from build123d import *

# Parameters (mm, degrees)
DODANIE_WYCI_GNI_CIE1_DEPTH = 40
ZAOKR_GLENIE1_R             = 20
SZKIC2_R                    = 12
WYTNIJ_WYCI_GNI_CIE1_DEPTH  = 725.630250542
SZKIC3_R                    = 8.15
WYTNIJ_WYCI_GNI_CIE2_DEPTH  = 725.630250542
SZKIC5_R                    = 14
DODANIE_WYCI_GNI_CIE2_DEPTH = 40
SZKIC6_W                    = 20
SZKIC6_H                    = 55
WYTNIJ_WYCI_GNI_CIE4_DEPTH  = 778.890737829
SZKIC4_R                    = 1.65
WYTNIJ_WYCI_GNI_CIE5_DEPTH  = 10
SFAZOWANIE1_SIZE            = 0.5
SFAZOWANIE2_SIZE            = 1


with BuildPart() as part:
    # Szkic1 → Dodanie-wyciągnięcie1 (new body)
    with BuildSketch(Plane.XY):
        Polygon((0, 0), (30, 0), (30, 670), (153, 670), (153, 0), (183, 0), (183, 700), (110, 700), (30, 700), (0, 700), align=None)
    extrude(amount=DODANIE_WYCI_GNI_CIE1_DEPTH)

    # Zaokrąglenie1
    zaokr_glenie1_edges = [part.edges().sort_by_distance(p)[0] for p in [
        (168, 0, 0),
        (168, 0, 40),
        (15, 0, 0),
        (15, 0, 40),
    ]]
    fillet(zaokr_glenie1_edges, radius=ZAOKR_GLENIE1_R - 0.0001)  # a hair under: the kernel refuses the full size

    # Szkic2 → Wytnij-wyciągnięcie1 (cut, through all)
    with BuildSketch(Plane.ZY):
        with Locations((20, 20)):
            Circle(SZKIC2_R)
    extrude(amount=-WYTNIJ_WYCI_GNI_CIE1_DEPTH, mode=Mode.SUBTRACT)

    # Szkic3 → Wytnij-wyciągnięcie2 (cut, through all)
    with BuildSketch(Plane(origin=(183, 0, 0), x_dir=(0, 0, -1), z_dir=(1, 0, 0))):
        with Locations(Location((-20, 70, 0), (0, 0, 90))):
            Circle(SZKIC3_R)
    extrude(amount=-WYTNIJ_WYCI_GNI_CIE2_DEPTH, mode=Mode.SUBTRACT)

    # Szkic5 → Dodanie-wyciągnięcie2 (add)
    with BuildSketch(Plane(origin=(0, 0, 0), x_dir=(-1, 0, 0), z_dir=(0, 0, -1))):
        with BuildLine():
            Line((-183, 700), (0, 700))
            Line((0, 700), (-74.84618459, 749.952964399))
            ThreePointArc((-74.84618459, 749.952964399), (-91.5, 755), (-108.15381541, 749.952964399))
            Line((-108.15381541, 749.952964399), (-183, 700))
        make_face()
        with Locations((-91.5, 725)):
            Circle(SZKIC5_R, mode=Mode.SUBTRACT)
    extrude(amount=-DODANIE_WYCI_GNI_CIE2_DEPTH)

    # Szkic6 → Wytnij-wyciągnięcie4 (cut, through all)
    with BuildSketch(Plane(origin=(183, 0, 0), x_dir=(0, 0, -1), z_dir=(1, 0, 0))):
        with Locations((-20, 727.5)):
            Rectangle(SZKIC6_W, SZKIC6_H)
    extrude(amount=-WYTNIJ_WYCI_GNI_CIE4_DEPTH, mode=Mode.SUBTRACT)

    # Szkic4 → Wytnij-wyciągnięcie5 (cut)
    with BuildSketch(Plane.ZY.offset(-153)):
        with Locations(Location((20, 657.5, 0), (0, 0, 270))):
            Circle(SZKIC4_R)
        with Locations(Location((20, 597.5, 0), (0, 0, 270))):
            Circle(SZKIC4_R)
        with Locations(Location((20, 537.5, 0), (0, 0, 270))):
            Circle(SZKIC4_R)
        with Locations(Location((20, 477.5, 0), (0, 0, 270))):
            Circle(SZKIC4_R)
        with Locations(Location((20, 417.5, 0), (0, 0, 270))):
            Circle(SZKIC4_R)
    extrude(amount=-WYTNIJ_WYCI_GNI_CIE5_DEPTH, mode=Mode.SUBTRACT)

    # Sfazowanie1
    sfazowanie1_edges = [part.edges().sort_by_distance(p)[0] for p in [
        (153, 659.15, 20),
        (153, 599.15, 20),
        (153, 539.15, 20),
        (153, 479.15, 20),
        (153, 419.15, 20),
    ]]
    chamfer(sfazowanie1_edges, length=SFAZOWANIE1_SIZE)

    # Sfazowanie2
    sfazowanie2_edges = [part.edges().sort_by_distance(p)[0] for p in [
        (30, 20, 8),
        (183, 20, 8),
        (153, 20, 8),
        (0, 20, 8),
        (0, 61.85, 20),
        (30, 61.85, 20),
        (153, 61.85, 20),
        (183, 61.85, 20),
    ]]
    chamfer(sfazowanie2_edges, length=SFAZOWANIE2_SIZE)


solid = part.part
Check sheet for the modelled part. Datum: model origin and axes. Units: mm. A direction names the side the tool comes from. Give positions to 0.01 mm unless a question says otherwise; leave off trailing zeros. Write each loop counter-clockwise with the first axis right and the second up, starting at its lowest first coordinate (ties: lowest second). Pieces come first, ordered by that corner, then holes. Notation, with made-up numbers: (-2.5, 5.25) -> (4.5, 5.25) arc R30 cw to (4.5, 27.25) -> close; hole circle Ø5 at (-29, 71.25). An arc over 180 degrees is marked (long way). Use one line per item in the form item = value. Start each with the question number.
1. Mould release check, pull along Y, two halves, no side actions. Record for faces 1 (the flat face through (0, 355, 20)), 2 (the cylindrical face through (168.2, 77.53, 16.88)), 3 (the cylindrical face through (14.804, 8.285, 17.399)), 4 (the flat face through (36.899, 724.627, 34.93)): pulls with the +Y half, pulls with the -Y half, needs draft (parallel to the pull), parting line crosses it, or undercut.
2. Section check A-A (y = 113.5). Record the cut outline in (x, z).
3. Go/stop test with flat-tipped pins: P1, Ø16, axis at x = 70, z = 20, coming from the +Y side; P2, Ø17, axis at x = 91.5, y = 725, coming from the +Z side; P3, Ø10, axis at x = 157, z = 6, coming from the -Y side; P4, Ø20, axis at x = 62, z = 24.5, coming from the -Y side. Record where each tip stops, or that it passes through.
4. Access from +Z, -Z, +X, -X, +Y, -Y to the whole of each face (thin tool, end or side, straight path). Record for faces 5 (the cylindrical face through (168.21, 5.703, 6.014)), 6 (the flat face through (91, 670, 20)).
5. Section check C-C (x = 138). Record the cut outline in (y, z), and give its area (3 significant figures).
6. Section check B-B (x = 95). Record the cut outline in (y, z), and give its area (3 significant figures).
7. Thickness scan on line 1 along X through (y, z) = (578, 23); line 2 along Z through (x, y) = (159, 597.5); line 3 along Z through (x, y) = (165.5, 70). Record the ranges inside material, lowest first. Write a range as from..to.
Conclusion:
q1.face_1 = needs draft
q1.face_2 = undercut
q1.face_3 = undercut
q1.face_4 = pulls with the +Y half
q2.outline = (0, 0) -> (30, 0) -> (30, 40) -> (0, 40) -> close; (153, 0) -> (183, 0) -> (183, 40) -> (153, 40) -> close
q3.P1 = 700
q3.P2 = through
q3.P3 = 2.14
q3.P4 = 670
q4.face_5 = -Z, +X, -X, -Y
q4.face_6 = +Z, -Z, -Y
q5.outline = (670, 0) -> (730.03, 0) -> (730.03, 10) -> (700, 10) -> (700, 30) -> (730.03, 30) -> (730.03, 40) -> (670, 40) -> close
q5.area = 1,800 mm²
q6.outline = (670, 0) -> (711.44, 0) -> (711.44, 10) -> (700, 10) -> (700, 30) -> (711.44, 30) -> (711.44, 40) -> (670, 40) -> close; (738.56, 0) -> (754.8, 0) -> (754.8, 10) -> (738.56, 10) -> close; (738.56, 30) -> (754.8, 30) -> (754.8, 40) -> (738.56, 40) -> close
q6.area = 1,750 mm²
q7.line_1 = 0..30, 153..183
q7.line_2 = 0..18.35, 21.65..40
q7.line_3 = 0..11.85, 28.15..40
